The model under review builds one solid part; all positions refer to its coordinate system, in mm. Face numbers are marked on the shaded views. A direction names the side the tool comes from. Give positions to 0.01 mm unless a question says otherwise; leave off trailing zeros. Order: outer loops, then holes, each group sorted by start corner. A loop starts at its lowest first (then second) coordinate and runs counter-clockwise, first axis right, second up. Notation, with made-up numbers: (57.5, 15.25) - (74.5, 15.25) arc R30 cw to (74.5, 45.25) - close; hole circle Ø11 at (-34, 3.25). An arc over 180 degrees is marked (long way). Write item = value, one per line. Start each with the question number.
1. We need section B-B, the plane x = -130.75. Give the boundary of the cut face in (y, z).
2. Machinability: for the marked faces 4, 5 and 6, which of the approach directions +Z, -Z, +X, -X, +Y, -Y give a long, thin tool a straight path to every point of the face, cutting with its end or side? Answer none if there is none.
3. We need section A-A, the plane z = 15.75. Give the boundary of the cut face in (x, y), and give its area (3 significant figures).
4. Mouldability with a two-part tool opening along Y and no side actions: class the marked faces 1, 2 and 3 as pulls with the +Y half, pulls with the -Y half, needs draft (parallel to the pull), parting line crosses it, or undercut.
5. We need section D-D, the plane y = 50.5. Give the boundary of the cut face in (x, z).
6. Wall thickness on probe 1 along Y at (x, z) = (-133.5, 20.25); probe 2 along Z at (x, y) = (-128.75, 49); probe 3 along Z at (x, y) = (-137, 34.25): over which ranges is each line inside the solid? List them lowest first.
7. For P1, Ø8, axis at x = -132.5, y = 40, coming from the -Z side; P2, Ø5.5, axis at x = -136, z = 19, coming from the -Y side; P3, Ø1, axis at y = 47, z = 19, coming from the +X side; P4, Ø6, axis at y = 37.5, z = 17, coming from the -X side, all flat-tipped, find the tip position at first contact; note any pin that passes through.
8. We need section C-C, the plane x = -135.75. State how many separate pieces and enclosed holes the cut face has, and give its area (3 significant figures).
from build123d import *

# Parameters (mm, degrees)
SKETCH_1_W      = 15
SKETCH_1_H      = 21
EXTRUDE_1_DEPTH = 2
SKETCH_2_W      = 12.5
SKETCH_2_H      = 19
EXTRUDE_2_DEPTH = 12.5
SKETCH_3_W      = 5
SKETCH_3_H      = 0.8
EXTRUDE_3_DEPTH = 7.5
CHAMFER_1_SIZE  = 1
EXTRUDE_START   = -2
EXTRUDE_4_DEPTH = 11
EXTRUDE_START_2 = -3.5
EXTRUDE_5_DEPTH = 5


with BuildPart() as part:
    # Эскиз1 → Бобышка-Вытянуть1 (new body)
    with BuildSketch(Plane.XY):
        with Locations((-135.472114918, 42.369501341)):
            Rectangle(SKETCH_1_W, SKETCH_1_H)
    extrude(amount=EXTRUDE_1_DEPTH)

    # Эскиз2 → Бобышка-Вытянуть2 (add)
    with BuildSketch(Plane.XY.offset(2)):
        with Locations((-135.472114918, 42.369501341)):
            Rectangle(SKETCH_2_W, SKETCH_2_H)
    extrude(amount=EXTRUDE_2_DEPTH)

    # Эскиз3 → Бобышка-Вытянуть3 (add)
    with BuildSketch(Plane.XY.offset(14.5)):
        with Locations((-135.472114918, 49.469501341)):
            Rectangle(SKETCH_3_W, SKETCH_3_H)
        with Locations((-135.472114918, 42.469501341)):
            Rectangle(SKETCH_3_W, SKETCH_3_H)
        with Locations((-135.472114918, 35.469501341)):
            Rectangle(SKETCH_3_W, SKETCH_3_H)
    extrude(amount=EXTRUDE_3_DEPTH)

    # Фаска1
    chamfer_1_edges = [part.edges().sort_by_distance(p)[0] for p in [
        (-132.972114918, 49.469501341, 22),
        (-137.972114918, 49.469501341, 22),
        (-132.972114918, 42.469501341, 22),
        (-137.972114918, 42.469501341, 22),
        (-132.972114918, 35.469501341, 22),
        (-137.972114918, 35.469501341, 22),
    ]]
    chamfer(chamfer_1_edges, length=CHAMFER_1_SIZE)

    # Эскиз5 → Бобышка-Вытянуть4 (add)
    with BuildSketch(Plane(origin=(-127.972114918, 0, 0), x_dir=(0, 0, -1), z_dir=(1, 0, 0)).offset(EXTRUDE_START)):
        with BuildLine():
            Line((0, 49.869501341), (0, 34.869501341))
            Line((0, 34.869501341), (0.354216836, 34.869501341))
            ThreePointArc((0.354216836, 34.869501341), (1.36091461, 42.154293323), (3.8, 49.092052117))
            ThreePointArc((3.8, 49.092052117), (1.929874617, 49.626797257), (0, 49.869501341))
        make_face()
    extrude(amount=-EXTRUDE_4_DEPTH)

    # Эскиз6 → Бобышка-Вытянуть5 (add)
    with BuildSketch(Plane(origin=(-129.222114918, 0, 0), x_dir=(0, 0, -1), z_dir=(1, 0, 0)).offset(EXTRUDE_START_2)):
        Polygon((-2, 51.869501341), (-2, 52.169501341), (-7.615330186, 52.869501341), (-12.960465763, 51.869501341), (-11.35692509, 51.869501341), (-7.615330186, 52.569501341), align=None)
        Polygon((-12.960465763, 32.869501341), (-11.35692509, 32.869501341), (-7.615330186, 32.169501341), (-2, 32.869501341), (-2, 32.569501341), (-7.615330186, 31.869501341), align=None)
    extrude(amount=-EXTRUDE_5_DEPTH)


solid = part.part
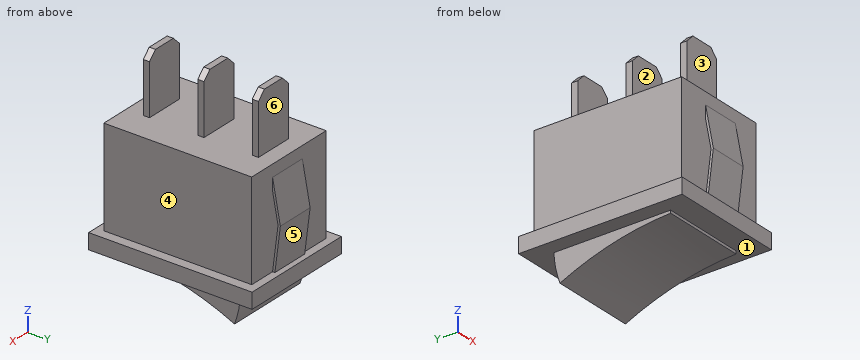
Model answer:
q1.outline = (31.87, 0) - (34.87, 0) - (34.87, -0.35) arc R36.69 cw to (49.09, -3.8) arc R12.69 ccw to (49.87, 0) - (52.87, 0) - (52.87, 2) - (51.87, 2) - (51.87, 14.5) - (32.87, 14.5) - (32.87, 2) - (31.87, 2) - close
q2.face_4 = +Z, +X, +Y, -Y
q2.face_5 = +X, -X, +Y
q2.face_6 = +Z, +X, -X, +Y
q3.outline = (-137.97, 35.07) - (-132.97, 35.07) - (-132.97, 35.87) - (-137.97, 35.87) - close; (-137.97, 42.07) - (-132.97, 42.07) - (-132.97, 42.87) - (-137.97, 42.87) - close; (-137.97, 49.07) - (-132.97, 49.07) - (-132.97, 49.87) - (-137.97, 49.87) - close
q3.area = 12.0 mm2
q4.face_1 = needs draft
q4.face_2 = undercut
q4.face_3 = pulls with the -Y half
q5.outline = (-142.97, 0) - (-127.97, 0) - (-127.97, 2) - (-129.22, 2) - (-129.22, 14.5) - (-141.72, 14.5) - (-141.72, 2) - (-142.97, 2) - close
q6.probe_1 = 35.07 to 35.87, 42.07 to 42.87, 49.07 to 49.87
q6.probe_2 = 0 to 2
q6.probe_3 = 0 to 14.5
q7.P1 = -1.86
q7.P2 = 35.07
q7.P3 = through
q7.P4 = -141.72
q8.separate_pieces = 1
q8.enclosed_holes = 2
q8.area = 328 mm2
